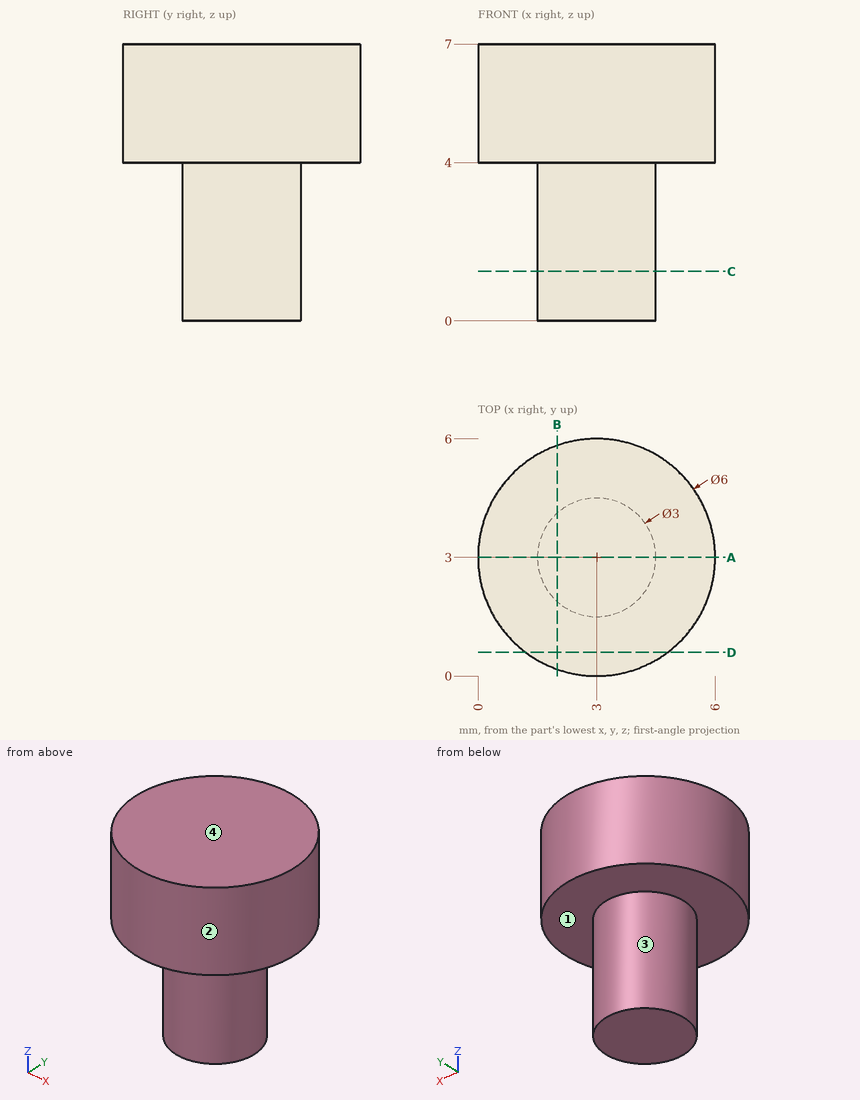
Source: three-view drawing plus pictorial views. Frame: mm from the lowest corner of the part. A direction names the side the tool comes from. Round coordinates to 2 decimals unless told otherwise and drop trailing zeros. Loops run counter-clockwise (first coordinate to the right, second up) from the corner with the lowest first, then second, coordinate; pieces in that order, holes last.
Item 1: Mould query, pull axis X, two halves, no side actions, for the marked faces 1 and 2. Classes: released by +X, released by -X, zero draft, split by the parting line, or undercut.
Checked values:
face 1: zero draft
face 2: split by the parting line
Item 2: Section D-D, the plane y = 0.6. Output: boundary loops of the cut face in (x, z).
Checked values:
outline: (1.2, 4) - (4.8, 4) - (4.8, 7) - (1.2, 7) - close
Item 3: Reachability of the marked faces 3 and 4 from +Z, -Z, +X, -X, +Y, -Y: full face, straight path, thin tool, end or side. Return the list, or none.
Checked values:
face 3: -Z
face 4: +Z, +X, -X, +Y, -Y
Item 4: Contact query for flat-ended pins moving along their axis: P1, Ø2, axis at x = 3.5, z = 2.5, coming from the +Y side; P2, Ø1, axis at x = 5, z = 4.5, coming from the +Y side; P3, Ø1.5, axis at x = 1.5, z = 1.5, coming from the +Y side. Output: stop coordinate, or through.
Checked values:
P1: stops at y = 4.5
P2: stops at y = 5.6
P3: stops at y = 4.3
Item 5: Section C-C, the plane z = 1.25. Output: boundary loops of the cut face in (x, y).
Checked values:
outline: circle Ø3 at (3, 3)
Item 6: Section B-B, the plane x = 2. Output: boundary loops of the cut face in (y, z).
Checked values:
outline: (0.17, 4) - (1.88, 4) - (1.88, 0) - (4.12, 0) - (4.12, 4) - (5.83, 4) - (5.83, 7) - (0.17, 7) - close
Item 7: Line query: L1, parallel to Z at x = 5.5, y = 3; L2, parallel to Y at x = 3, z = 1; L3, parallel to Y at x = 1.75, z = 0.5. Output: solid intervals per line, ascending.
Checked values:
L1: z = 4 to 7
L2: y = 1.5 to 4.5
L3: y = 2.17 to 3.83
Item 8: Section A-A, the plane y = 3. Output: boundary loops of the cut face in (x, z).
Checked values:
outline: (0, 4) - (1.5, 4) - (1.5, 0) - (4.5, 0) - (4.5, 4) - (6, 4) - (6, 7) - (0, 7) - close
